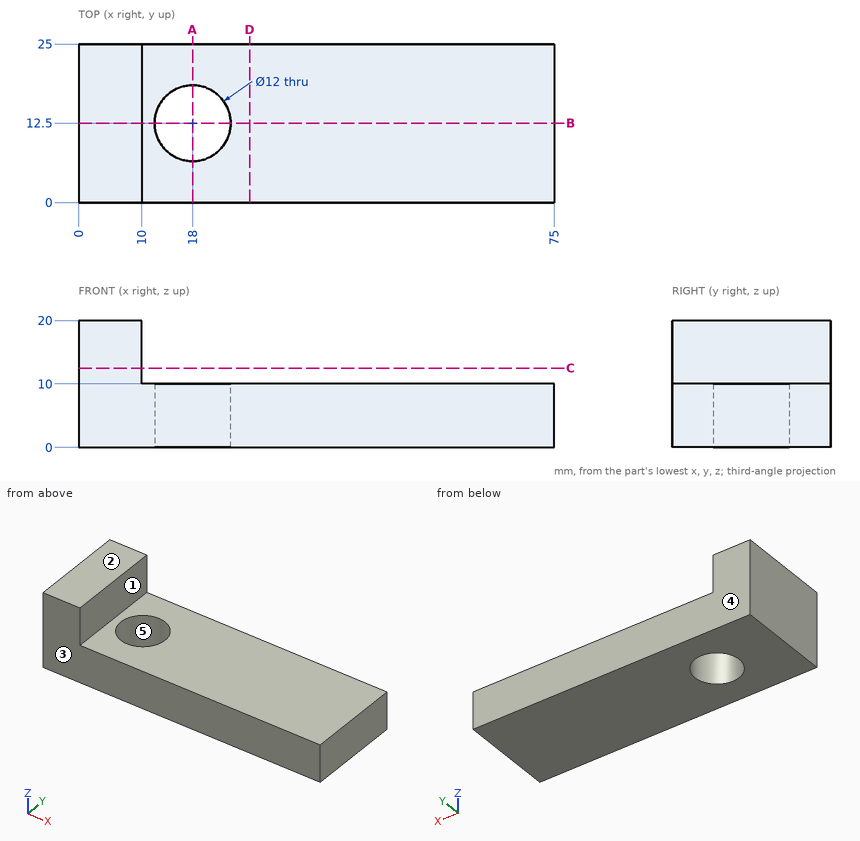
Part print with two shaded views. Sizes in mm from the minimum x, y, z corner. A direction names the side the tool comes from. Round coordinates to 2 decimals unless told otherwise and drop trailing zeros. Order: outer loops, then holes, each group sorted by start corner. A loop starts at its lowest first (then second) coordinate and runs counter-clockwise, first axis right, second up. Notation, with made-up numbers: M 3.5,-20 L 29.5,-20 A15 cw 29.5,6 Z; hole C 19.25,77 d4. An arc over 180 degrees is marked long. Answer in a Markdown table with one row per item. Add a question column.
Q1. 3-axis set-ups, long thin cutter, end or side, ignore diameter. For the marked faces 1 and 2: which of +Z, -Z, +X, -X, +Y, -Y reach the whole face in a straight line?
Q2. Cut at C-C on z = 12.5. Give the cut face in (x, y), and give its area (3 significant figures).
Q3. Mould opens along Y. For the marked faces 3, 4 and 5 say: +Y half, -Y half, draft (parallel to the pull), parting line (faces both ways), or undercut.
Q4. Cut at A-A on x = 18. Give the cut face in (y, z).
Q5. Cut at D-D on x = 27. Give the cut face in (y, z), and give its area (3 significant figures).
Q6. Cut at B-B on y = 12.5. Give the cut face in (x, z), and give its area (3 significant figures).
Q7. Pin check, flat tip, straight feed: pin 1 (3 mm diameter, centred on y = 14.5, z = 13.5, fed in from +X). Stop position of the tip, or through.
Q8. Wall check: L1, parallel to Y at x = 18, z = 4; L2, parallel to X at y = 12.5, z = 3; L3, parallel to Z at x = 20.5, y = 3.75. Give the ranges that are in metal, low to high. Write a range as from..to.
Established:
| question | item | result |
|---|---|---|
| 1 | face 1 | +Z, +X, +Y, -Y |
| 1 | face 2 | +Z, +X, -X, +Y, -Y |
| 2 | outline | M 0,0 L 10,0 L 10,25 L 0,25 Z |
| 2 | area | 250 mm2 |
| 3 | face 3 | -Y half |
| 3 | face 4 | +Y half |
| 3 | face 5 | undercut |
| 4 | outline | M 0,0 L 6.5,0 L 6.5,10 L 0,10 Z; M 18.5,0 L 25,0 L 25,10 L 18.5,10 Z |
| 5 | outline | M 0,0 L 25,0 L 25,10 L 0,10 Z |
| 5 | area | 250 mm2 |
| 6 | outline | M 0,0 L 12,0 L 12,10 L 10,10 L 10,20 L 0,20 Z; M 24,0 L 75,0 L 75,10 L 24,10 Z |
| 6 | area | 730 mm2 |
| 7 | pin 1 | stops at x = 10 |
| 8 | L1 | y = 0..6.5, 18.5..25 |
| 8 | L2 | x = 0..12, 24..75 |
| 8 | L3 | z = 0..10 |
